Autodesk Inventor part; units mm, degrees
ref_plane "Work Plane1" through (0, 0, 13.5128) normal (0, 0, 1) x (1, 0, 0)
ref_plane "YZ Plane" through (0, 0, 0) normal (1, 0, 0) x (0, 1, 0)
ref_plane "XZ Plane" through (0, 0, 0) normal (0, 1, 0) x (-1, 0, 0)
sketch "Sketch1" plane through (0, 0, 0) normal (0, 0, 1) x (1, 0, 0)
  line L0 (-12.7, 5.08) -> (12.7, 5.08)
  line L1 (12.7, 5.08) -> (12.7, -5.08)
  line L2 (12.7, -5.08) -> (-12.7, -5.08)
  line L3 (-12.7, -5.08) -> (-12.7, 5.08)
  point P0 (0, 0)
  point P1 (0, 5.08)
  point P2 (-12.7, 0)
  dimension "d0" = 25.4
  dimension "d1" = 10.16
extrude "Extrusion1" add sketch "Sketch1" along normal blind 0.8128
ref_plane "Work Plane1" through (0, 0, 13.5128) normal (0, 0, 1) x (1, 0, 0)
sketch "Sketch2" plane through (0, 0, 13.5128) normal (0, 0, 1) x (1, 0, 0)
  line L0 (12.7, 5.08) -> (12.7, -5.08)
  line L1 (-12.7, 5.08) -> (12.7, 5.08)
  line L2 (-12.7, -5.08) -> (-12.7, 5.08)
  line L3 (12.7, -5.08) -> (-12.7, -5.08)
  line L4 (-3.3655, 3.556) -> (3.3655, 3.556)
  line L5 (-3.3655, -3.556) -> (3.3655, -3.556)
  line L6 (-4.953, 1.9685) -> (-4.953, -1.9685)
  line L7 (4.953, 1.9685) -> (4.953, -1.9685)
  arc A0 (-3.3655, 3.556) -> (-4.953, 1.9685) centre (-3.3655, 1.9685) ccw
  arc A1 (-4.953, -1.9685) -> (-3.3655, -3.556) centre (-3.3655, -1.9685) ccw
  arc A2 (3.3655, -3.556) -> (4.953, -1.9685) centre (3.3655, -1.9685) ccw
  arc A3 (4.953, 1.9685) -> (3.3655, 3.556) centre (3.3655, 1.9685) ccw
  point P0 (0, 0)
  point P1 (0, 3.556)
  point P2 (0, -3.556)
  point P3 (-4.953, 0)
  point P4 (4.953, 0)
  dimension "d5" = 6.731
  dimension "d6" = 6.731
  dimension "d7" = 3.937
  dimension "d8" = 3.937
  dimension "d9" = 4.953
  dimension "d10" = 4.953
  dimension "d11" = 3.556
  dimension "d12" = 3.556
  dimension "d13" = 1.5875
  dimension "d14" = 1.5875
  dimension "d15" = 1.5875
  dimension "d16" = 1.5875
extrude "Extrusion2" cut sketch "Sketch2" against normal blind 25.4 contours L4 A3 L7 A2 L5 A1 L6 A0
sketch "Sketch3" plane through (0, 0, 13.5128) normal (0, 0, 1) x (1, 0, 0)
  arc A0 (-3.3655, 3.556) -> (-4.953, 1.9685) centre (-3.3655, 1.9685) ccw
  line L0 (-3.3655, 3.556) -> (3.3655, 3.556)
  arc A1 (4.953, 1.9685) -> (3.3655, 3.556) centre (3.3655, 1.9685) ccw
  line L1 (4.953, 1.9685) -> (4.953, -1.9685)
  arc A2 (3.3655, -3.556) -> (4.953, -1.9685) centre (3.3655, -1.9685) ccw
  line L2 (3.3655, -3.556) -> (-3.3655, -3.556)
  arc A3 (-4.953, -1.9685) -> (-3.3655, -3.556) centre (-3.3655, -1.9685) ccw
  line L3 (-4.953, -1.9685) -> (-4.953, 1.9685)
  line L4 (12.7, 5.08) -> (12.7, -5.08)
  line L5 (-12.7, 5.08) -> (12.7, 5.08)
  line L6 (-12.7, -5.08) -> (-12.7, 5.08)
  line L7 (12.7, -5.08) -> (-12.7, -5.08)
  line L8 (-12.7, 1.5875) -> (-8.128, 1.5875)
  line L9 (-12.7, -1.5875) -> (-8.128, -1.5875)
  arc A4 (-8.128, -1.5875) -> (-8.128, 1.5875) centre (-8.128, 0) ccw
  point P0 (0, 0)
  dimension "d19" = 4.572
  dimension "d20" = 3.4925
  dimension "d21" = 4.572
  dimension "d22" = 3.175
  dimension "d24" = 1.5875
extrude "Extrusion3" cut sketch "Sketch3" against normal blind 25.4 contours L8 A4 L9 L6
mirror "Mirror1" about plane through (0, 0, 0) normal (1, 0, 0) of "Extrusion3"
sketch "Sketch5" plane through (0, 0, 0.8128) normal (0, 0, 1) x (1, 0, 0)
  line L0 (4.953, 1.9685) -> (4.953, -1.9685) construction
  line L1 (-4.953, -1.9685) -> (4.953, -1.9685)
  line L2 (4.953, -1.9685) -> (4.953, 7.0011)
  line L3 (4.953, 7.0011) -> (-4.953, 7.0011)
  line L4 (-4.953, 7.0011) -> (-4.953, -1.9685)
  point P0 (0, 0)
extrude "Extrusion5" cut sketch "Sketch5" against normal blind 25.4
fillet "Fillet1" radius 1.524 2 edges at (-4.953, 5.08, 0.4064) (4.953, 5.08, 0.4064)
sketch "Sketch6" plane through (0, 0, 0.8128) normal (0, 0, 1) x (1, 0, 0)
  arc A0 (6.477, 5.08) -> (4.953, 3.556) centre (6.477, 3.556) ccw construction
  line L0 (4.953, 3.556) -> (4.953, -1.9685) construction
  arc A1 (3.3655, -3.556) -> (4.953, -1.9685) centre (3.3655, -1.9685) ccw construction
  line L1 (3.3655, -3.556) -> (-3.3655, -3.556) construction
  arc A2 (-4.953, -1.9685) -> (-3.3655, -3.556) centre (-3.3655, -1.9685) ccw construction
  line L2 (-4.953, -1.9685) -> (-4.953, 3.556) construction
  arc A3 (-4.953, 3.556) -> (-6.477, 5.08) centre (-6.477, 3.556) ccw construction
  line L3 (-12.7, 5.08) -> (-6.477, 5.08) construction
  line L4 (-12.7, 1.5875) -> (-12.7, 5.08) construction
  line L5 (-12.7, 1.5875) -> (-8.128, 1.5875) construction
  arc A4 (-8.128, -1.5875) -> (-8.128, 1.5875) centre (-8.128, 0) ccw construction
  line L6 (-8.128, -1.5875) -> (-12.7, -1.5875) construction
  line L7 (-12.7, -5.08) -> (-12.7, -1.5875) construction
  line L8 (12.7, -5.08) -> (-12.7, -5.08) construction
  line L9 (12.7, -1.5875) -> (12.7, -5.08) construction
  line L10 (12.7, -1.5875) -> (8.128, -1.5875) construction
  arc A5 (8.128, 1.5875) -> (8.128, -1.5875) centre (8.128, 0) ccw construction
  line L11 (8.128, 1.5875) -> (12.7, 1.5875) construction
  line L12 (12.7, 5.08) -> (12.7, 1.5875) construction
  line L13 (6.477, 5.08) -> (12.7, 5.08) construction
  point P0 (0, 0)
properties part number "headplate_largerCenter_frontcutout"
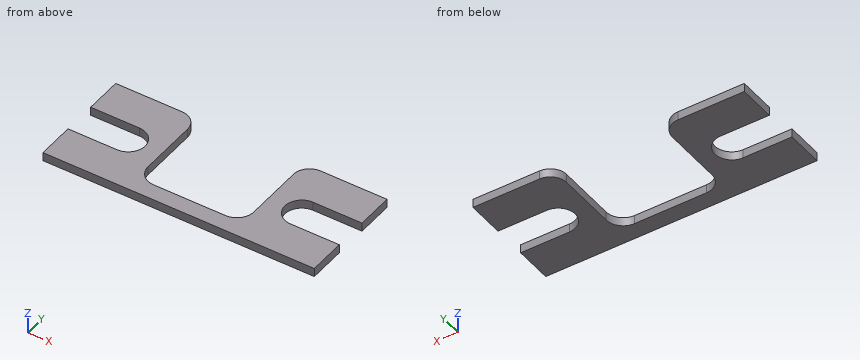
The model under review builds one solid part; all positions refer to its coordinate system, in mm. Give positions to 0.01 mm unless a question says otherwise; leave off trailing zeros. Loops run counter-clockwise (first coordinate to the right, second up) from the corner with the lowest first, then second, coordinate; pieces in that order, holes last. Notation, with made-up numbers: (56.25, 88.25) -> (94.25, 88.25) arc R14 cw to (94.25, 107.25) -> close; hole circle Ø2 at (82, 80). An arc over 180 degrees is marked (long way). Answer as a JSON object with one key per item and string values. Group by question number.
Q1. Take a section at C-C (z = 0.65). Write out the cut boundary in (x, y) (1 decimal).
Q2. Take a section at B-B (y = 0). Write out the cut boundary in (x, z).
Q3. Wall thickness on line 1 along Y through (x, z) = (10.25, 0.55); line 2 along X through (y, z) = (3, 0.75); line 3 along X through (y, z) = (-1, 0.35): over which ranges is each line inside the solid? List them lowest first.
Q4. Take a section at D-D (x = -2.5). Write out the cut boundary in (y, z), plus the area to 3 significant figures.
Q5. Insertion check: pin 1 (1.5 mm diameter, centred on x = 3.5, y = 3.5, fed in from +Z). The pin has a flat end and moves straight along its axis. Give the tip position at first contact, or say it passes through.
Q6. Take a section at A-A (x = -10.75). Write out the cut boundary in (y, z).
Answer below:
{
 "1": {"outline": "(-12.7, -5.1) -> (12.7, -5.1) -> (12.7, -1.6) -> (8.1, -1.6) arc R1.6 cw to (8.1, 1.6) -> (12.7, 1.6) -> (12.7, 5.1) -> (6.5, 5.1) arc R1.5 ccw to (5, 3.6) -> (5, -2) arc R1.6 cw to (3.4, -3.6) -> (-3.4, -3.6) arc R1.6 cw to (-5, -2) -> (-5, 3.6) arc R1.5 ccw to (-6.5, 5.1) -> (-12.7, 5.1) -> (-12.7, 1.6) -> (-8.1, 1.6) arc R1.6 cw to (-8.1, -1.6) -> (-12.7, -1.6) -> close"},
 "2": {"outline": "(-6.54, 0) -> (-4.95, 0) -> (-4.95, 0.81) -> (-6.54, 0.81) -> close; (4.95, 0) -> (6.54, 0) -> (6.54, 0.81) -> (4.95, 0.81) -> close"},
 "3": {"line 1": "y = -5.08 to -1.59, 1.59 to 5.08", "line 2": "x = -12.7 to -4.95, 4.95 to 12.7", "line 3": "x = -6.9 to -4.95, 4.95 to 6.9"},
 "4": {"outline": "(-5.08, 0) -> (-3.56, 0) -> (-3.56, 0.81) -> (-5.08, 0.81) -> close", "area": "1.24 mm2"},
 "5": {"pin 1": "passes through"},
 "6": {"outline": "(-5.08, 0) -> (-1.59, 0) -> (-1.59, 0.81) -> (-5.08, 0.81) -> close; (1.59, 0) -> (5.08, 0) -> (5.08, 0.81) -> (1.59, 0.81) -> close"}
}
